from build123d import *

# Parameters (mm, degrees)
F3_DEPTH = 4


with BuildPart() as f1:
    # F0 (on Front) → F1 (revolve)
    with BuildSketch(Plane.XZ):
        with BuildLine():
            Line((12, 9), (12, 12))
            Line((12, 12), (3.1, 12))
            Line((3.1, 12), (3.1, 0))
            Line((3.1, 0), (12, 0))
            Line((12, 0), (12, 3))
            ThreePointArc((12, 3), (9.800525, 6), (12, 9))
        make_face()
    revolve(axis=Axis((0, 0, 8.473897), (0, 0, 1)))

    # F2 (on face) → F3 (cut)
    with BuildSketch(Plane.XY.offset(12)):
        with BuildLine():
            Line((-9, -0.85), (-2.981191, -0.85))
            ThreePointArc((-2.981191, -0.85), (-3.1, 0), (-2.981191, 0.85))
            Line((-2.981191, 0.85), (-9, 0.85))
            Line((-9, 0.85), (-9, -0.85))
        make_face()
        with BuildLine():
            Line((2.981191, -0.85), (9, -0.85))
            Line((9, -0.85), (9, 0.85))
            Line((9, 0.85), (2.981191, 0.85))
            ThreePointArc((2.981191, 0.85), (3.070154, 0.429132), (3.1, 0))
            ThreePointArc((3.1, 0), (3.070154, -0.429132), (2.981191, -0.85))
        make_face()
    extrude(amount=-F3_DEPTH, mode=Mode.SUBTRACT)


solid = f1.part
Design review of the part built by this model. Coordinates are the model's own, in mm. A direction names the side the tool comes from. Round coordinates to 2 decimals unless told otherwise and drop trailing zeros. Order: outer loops, then holes, each group sorted by start corner. A loop starts at its lowest first (then second) coordinate and runs counter-clockwise, first axis right, second up.
1) Draft analysis for pull direction X (two halves, no side actions). For faces 1 (the flat face through (-2.5, -2.5, 0)), 2 (the flat face through (6, 0, 8)), 3 (the cylindrical face through (-11.99, 0.53, 10.52)), state which applies: released by +X, released by -X, zero draft, split by the parting line, or undercut.
The answers:
face 1: zero draft
face 2: undercut
face 3: split by the parting line
2) Consider section A-A (y = 0). State the section outline as (x, z) points.
The answers:
outline: (-12, 0) - (-3.1, 0) - (-3.1, 8) - (-9, 8) - (-9, 12) - (-12, 12) - (-12, 9) arc R3.15 cw to (-12, 3) - close; (3.1, 0) - (12, 0) - (12, 3) arc R3.15 cw to (12, 9) - (12, 12) - (9, 12) - (9, 8) - (3.1, 8) - close
3) Consider section D-D (z = 1). State the section outline as (x, y) points, plus the area to 3 significant figures.
The answers:
outline: circle Ø24 at (0, 0); hole circle Ø6.2 at (0, 0)
area: 422 mm2
4) Machinability: for faces 4 (the flat face through (-6, -0.85, 10)), 5 (the cylindrical face through (2.957, 0.931, 5.916)), which of the approach directions +Z, -Z, +X, -X, +Y, -Y give a long, thin tool a straight path to every point of the face, cutting with its end or side? Answer none if there is none.
The answers:
face 4: +Z
face 5: +Z, -Z
5) For L1, parallel to Y at x = 0, z = 9.25; L2, parallel to Y at x = 0, z = 4.75; L3, parallel to Z at x = -10, y = 6, list the stretches that pass through material, from the lowest coordinate up.
The answers:
L1: y = -12 to -3.1, 3.1 to 12
L2: y = -10.06 to -3.1, 3.1 to 10.06
L3: z = 0 to 3.13, 8.87 to 12
6) Consider section B-B (x = 0). State the section outline as (y, z) points.
The answers:
outline: (-12, 0) - (-3.1, 0) - (-3.1, 12) - (-12, 12) - (-12, 9) arc R3.15 cw to (-12, 3) - close; (3.1, 0) - (12, 0) - (12, 3) arc R3.15 cw to (12, 9) - (12, 12) - (3.1, 12) - close
7) Consider section C-C (z = 11.25). State the section outline as (x, y) points.
The answers:
outline: circle Ø24 at (0, 0); hole (-9, -0.85) - (-2.98, -0.85) arc R3.1 ccw to (2.98, -0.85) - (9, -0.85) - (9, 0.85) - (2.98, 0.85) arc R3.1 ccw to (-2.98, 0.85) - (-9, 0.85) - close
8) Clearance check with flat-ended pins moving along their axes: pin 1 Ø0.8 at (x, y) = (-6, 0) entering from +Z; pin 2 Ø2 at (x, y) = (-3.5, 0.5) entering from -Z; pin 3 Ø6 at (y, z) = (8, 10.5) entering from +X; pin 4 Ø5.5 at (x, y) = (0, 0) entering from +Z. State where each tip first meets the part, or that it passes through.
The answers:
pin 1: stops at z = 8
pin 2: stops at z = 0
pin 3: stops at x = 10.91
pin 4: passes through
